Check sheet for the modelled part. Datum: model origin and axes. Units: mm. A direction names the side the tool comes from. Round coordinates to 2 decimals unless told otherwise and drop trailing zeros. Order: outer loops, then holes, each group sorted by start corner. A loop starts at its lowest first (then second) coordinate and runs counter-clockwise, first axis right, second up.
Q1. Cross-section at C-C on z = -117.5. Record the cut outline in (x, y), then the cut area to 3 significant figures.
Q2. Cross-section at A-A on y = 0. Record the cut outline in (x, z).
Q3. Scan lines: probe 1 along Y at (x, z) = (-4.5, -155.5); probe 2 along X at (y, z) = (0, -56.5); probe 3 along Y at (x, z) = (-11, -31). Record each from-to range of solid material in increasing order.
Q4. Depth check by flat-ended pin: P1, Ø8, axis at y = 241, z = -135.5, coming from the +X side; P2, Ø2, axis at y = 276.5, z = -108.5, coming from the +X side; P3, Ø2, axis at y = 29, z = -158.5, coming from the -X side. Enter the tip coordinate at first touch or a pass-through.
Q5. Set-up check for faces 4 (the cylindrical face through (-230.007, -299.968, -143.988)), 5 (the flat face through (212, -332, -244)): record each of +Z, -Z, +X, -X, +Y, -Y from which the full face is reachable in a straight line by a thin tool's end or side.
Q6. Mould release check, pull along Z, two halves, no side actions. Record for faces 1 (the flat face through (182, -332, -284)), 2 (the cylindrical face through (-155.117, 374.117, -264.28)), 3 (the flat face through (212, -332, -40)): +Z half, -Z half, draft (parallel to the pull), parting line (faces both ways), or undercut.
Autodesk Inventor part; units mm, degrees
ref_plane "YZ Plane" through (0, 0, 0) normal (1, 0, 0) x (0, 1, 0)
ref_plane "XZ Plane" through (0, 0, 0) normal (0, 1, 0) x (-1, 0, 0)
ref_plane "XY Plane" through (0, 0, 0) normal (0, 0, 1) x (1, 0, 0)
sketch "Sketch1" plane through (0, 0, 0) normal (1, 0, 0) x (0, 1, 0)
  line L0 (0, 0) -> (0, -284)
  line L1 (0, 0) -> (378, 0)
  line L2 (378, 0) -> (378, -284)
  line L3 (378, -284) -> (0, -284)
  line L4 (378, 0) -> (405, 0)
  line L5 (405, 0) -> (405, -40)
  line L6 (405, -40) -> (390, -40)
  line L7 (390, -40) -> (390, -244)
  line L8 (390, -244) -> (405, -244)
  line L9 (405, -244) -> (405, -284)
  line L10 (378, -284) -> (405, -284)
  dimension "d0" = 756
  dimension "d1" = 780
  dimension "d2" = 810
  dimension "d3" = 40
  dimension "d4" = 40
  dimension "d5" = 284
revolve "Revolution1" add sketch "Sketch1" angle 360 about axis through (0, 0, 0) along (0, 0, -1) contours L4 L5 L6 L7 L8 L9 L10 L2
properties part number "DiscoCorpoTurbina4" material "Steel, Alloy"
Results found:
1. outline: circle Ø780 at (0, 0); hole circle Ø756 at (0, 0)
1. area: 29,000 mm2
2. outline: (-405, -284) - (-378, -284) - (-378, 0) - (-405, 0) - (-405, -40) - (-390, -40) - (-390, -244) - (-405, -244) - close; (378, -284) - (405, -284) - (405, -244) - (390, -244) - (390, -40) - (405, -40) - (405, 0) - (378, 0) - close
3. probe 1: y = -389.97 to -377.97, 377.97 to 389.97
3. probe 2: x = -390 to -378, 378 to 390
3. probe 3: y = -404.85 to -377.84, 377.84 to 404.85
4. P1: stops at x = 309.73
4. P2: stops at x = 276.04
4. P3: stops at x = -388.99
5. face 4: +Z, -Z
5. face 5: none
6. face 1: -Z half
6. face 2: draft
6. face 3: undercut
